```python
from build123d import *

# Parameters (mm, degrees)
BOSS_EXTRUDE1_DEPTH     = 11.5
CUT_EXTRUDE2_DEPTH      = 20.579495528
CUT_EXTRUDE2_DEPTH_BACK = 20.579495528
SKETCH2_R               = 1.016


with BuildPart() as part:
    # Sketch1 → Boss-Extrude1 (new body)
    with BuildSketch(Plane.XY):
        with BuildLine():
            Line((7.5, 9.576744186), (0, 9.576744186))
            Line((0, 9.576744186), (0, 8.586804732))
            Line((0, 8.586804732), (4.625286285, 8.586804732))
            ThreePointArc((4.625286285, 8.586804732), (6.039499847, 8.001018294), (6.625286285, 6.586804732))
            Line((6.625286285, 6.586804732), (6.625286285, -1.923255814))
            Line((6.625286285, -1.923255814), (13.367366986, -1.923255814))
            Line((13.367366986, -1.923255814), (13.367366986, 1.066741541))
            Line((13.367366986, 1.066741541), (9.5, 1.066741541))
            ThreePointArc((9.5, 1.066741541), (8.085786438, 1.652527979), (7.5, 3.066741541))
            Line((7.5, 3.066741541), (7.5, 9.576744186))
        make_face()
        with BuildLine():
            Line((0, 9.576744186), (-7.5, 9.576744186))
            Line((-7.5, 9.576744186), (-7.5, 3.066741541))
            ThreePointArc((-7.5, 3.066741541), (-8.085786438, 1.652527979), (-9.5, 1.066741541))
            Line((-9.5, 1.066741541), (-13.367366986, 1.066741541))
            Line((-13.367366986, 1.066741541), (-13.367366986, -1.923255814))
            Line((-13.367366986, -1.923255814), (-6.625286285, -1.923255814))
            Line((-6.625286285, -1.923255814), (-6.625286285, 6.586804732))
            ThreePointArc((-6.625286285, 6.586804732), (-6.039499847, 8.001018294), (-4.625286285, 8.586804732))
            Line((-4.625286285, 8.586804732), (0, 8.586804732))
            Line((0, 8.586804732), (0, 9.576744186))
        make_face()
    extrude(amount=BOSS_EXTRUDE1_DEPTH)

    # Sketch2 → Cut-Extrude2 (cut, two sides: drawn at the far end of the back side and taken through both)
    with BuildSketch(Plane(origin=(0, 1.066741541, 0), x_dir=(1, 0, 0), z_dir=(0, 1, 0)).offset(-CUT_EXTRUDE2_DEPTH_BACK)):
        with Locations(Location((-9, -5.507720323, 0), (0, 0, 180))):
            Circle(SKETCH2_R)
        with Locations(Location((9, -5.507720323, 0), (0, 0, 180))):
            Circle(SKETCH2_R)
    extrude(amount=CUT_EXTRUDE2_DEPTH + CUT_EXTRUDE2_DEPTH_BACK, mode=Mode.SUBTRACT)


solid = part.part
```
The model under review builds one solid part; all positions refer to its coordinate system, in mm. A direction names the side the tool comes from. Round coordinates to 2 decimals unless told otherwise and drop trailing zeros. Write each loop counter-clockwise with the first axis right and the second up, starting at its lowest first coordinate (ties: lowest second). Pieces come first, ordered by that corner, then holes. Notation, with made-up numbers: M -17.5,83.5 L 24.5,83.5 A26 ccw 24.5,115.5 Z; hole C -29,-39 d10. An arc over 180 degrees is marked long. Use CSV: the item, a comma, the result in double quotes. Start each with the question number.
(1) We need section D-D, the plane x = -5. State the section outline as (y, z) points, then the cut area to 3 significant figures.
(2) Clearance check with flat-ended pins moving along their axes: P1, Ø2, axis at y = 6.5, z = 4, coming from the -X side; P2, Ø5, axis at y = 5.5, z = 7, coming from the +X side; P3, Ø2.5, axis at x = -9, z = 5.51, coming from the +Y side; P4, Ø1.8, axis at x = 9, z = 5.51, coming from the +Y side. State where each tip first meets the part, or that it passes through.
(3) We need section B-B, the plane x = -9. State the section outline as (y, z) points.
(4) For line 1 along Z through (x, y) = (-9, 0.7); line 2 along X through (y, z) = (3, 2.75); line 3 along X through (y, z) = (0, 2), list the stretches that pass through material, from the lowest coordinate up.
(5) Tool access review of faces 4 (the face through (-13.367, 0, 6)), 5 (the face through (-7.5, 6, 6)), 6 (the face through (13.367, 0, 6)), 7 (the face through (7.5, 6, 6)), 8 (the face through (6.02, 8.02, 5.67)): name each direction out of +Z, -Z, +X, -X, +Y, -Y from which nothing blocks a thin tool from reaching the whole face with its end or side.
(6) We need section C-C, the plane z = 9.25. State the section outline as (x, y) points, then the cut area to 3 significant figures.
(7) We need section A-A, the plane y = 3.75. State the section outline as (x, z) points, then the cut area to 3 significant figures.
(8) The part is to be moulded in two halves that separate along Z. For faces 1 (the face through (0, 9, 0)), 2 (the face through (-7.985, -0.516, 5.552)), 3 (the face through (11, 1.067, 6)), say which applies: +Z half, -Z half, draft (parallel to the pull), parting line (faces both ways), or undercut.
Findings:
1,outline,"M 8.55,0 L 9.58,0 L 9.58,11.5 L 8.55,11.5 Z"
1,area,"11.8 mm^2"
2,P1,"x = -7.5"
2,P2,"x = 7.5"
2,P3,"y = 2.1"
2,P4,"through"
3,outline,"M -1.92,0 L 1.13,0 L 1.13,4.49 L -1.92,4.49 Z; M -1.92,6.52 L 1.13,6.52 L 1.13,11.5 L -1.92,11.5 Z"
4,line 1,"0 to 4.49, 6.52 to 11.5"
4,line 2,"-7.5 to -6.63, 6.63 to 7.5"
4,line 3,"-13.37 to -6.63, 6.63 to 13.37"
5,face 4,"+Z, -Z, -X, +Y, -Y"
5,face 5,"+Z, -Z, -X, +Y"
5,face 6,"+Z, -Z, +X, +Y, -Y"
5,face 7,"+Z, -Z, +X, +Y"
5,face 8,"+Z, -Z, -Y"
6,outline,"M -13.37,-1.92 L -6.63,-1.92 L -6.63,6.59 A2 cw -4.63,8.59 L 4.63,8.59 A2 cw 6.63,6.59 L 6.63,-1.92 L 13.37,-1.92 L 13.37,1.07 L 9.5,1.07 A2 cw 7.5,3.07 L 7.5,9.58 L -7.5,9.58 L -7.5,3.07 A2 cw -9.5,1.07 L -13.37,1.07 Z"
6,area,"71.8 mm^2"
7,outline,"M -7.5,0 L -6.63,0 L -6.63,11.5 L -7.5,11.5 Z; M 6.63,0 L 7.5,0 L 7.5,11.5 L 6.63,11.5 Z"
7,area,"20.1 mm^2"
8,face 1,"-Z half"
8,face 2,"undercut"
8,face 3,"draft"
